Work out the finished part from the listing and answer in its coordinate system (mm). Round coordinates to 2 decimals unless told otherwise and drop trailing zeros. Answer in a Markdown table with one row per item.
```python
from build123d import *

# Parameters (mm, degrees)
MOTOR_AND_BATTERY_FLOOR_PROFILE_R   = 2.75
MOTOR_AND_BATTERY_FLOOR_PROFILE_R_2 = 1.75
MOTOR_AND_BATTERY_FLOOR_PROFILE_R_3 = 2.2
MOTOR_AND_BATTERY_FLOOR_DEPTH       = 2


with BuildPart() as part:
    # Motor and battery floor profile → Motor and battery floor (new body)
    with BuildSketch(Plane.XY):
        Polygon((-140, -143), (-94, -143), (-94, -104), (93, -104), (93, -143), (103, -143), (103, 143), (93, 143), (93, 104), (-94, 104), (-94, 143), (-140, 143), align=None)
        with Locations((-90, -91)):
            Circle(MOTOR_AND_BATTERY_FLOOR_PROFILE_R, mode=Mode.SUBTRACT)
        with Locations((-90, 91)):
            Circle(MOTOR_AND_BATTERY_FLOOR_PROFILE_R, mode=Mode.SUBTRACT)
        with Locations((-31, -91)):
            Circle(MOTOR_AND_BATTERY_FLOOR_PROFILE_R, mode=Mode.SUBTRACT)
        with Locations((-31, 91)):
            Circle(MOTOR_AND_BATTERY_FLOOR_PROFILE_R, mode=Mode.SUBTRACT)
        with Locations((31, -91)):
            Circle(MOTOR_AND_BATTERY_FLOOR_PROFILE_R, mode=Mode.SUBTRACT)
        with Locations((31, 91)):
            Circle(MOTOR_AND_BATTERY_FLOOR_PROFILE_R, mode=Mode.SUBTRACT)
        with Locations((90, -91)):
            Circle(MOTOR_AND_BATTERY_FLOOR_PROFILE_R, mode=Mode.SUBTRACT)
        with Locations((90, 91)):
            Circle(MOTOR_AND_BATTERY_FLOOR_PROFILE_R, mode=Mode.SUBTRACT)
        with Locations((-134, -108)):
            Circle(MOTOR_AND_BATTERY_FLOOR_PROFILE_R_2, mode=Mode.SUBTRACT)
        with Locations((-134, -17)):
            Circle(MOTOR_AND_BATTERY_FLOOR_PROFILE_R_2, mode=Mode.SUBTRACT)
        with Locations((-134, 17)):
            Circle(MOTOR_AND_BATTERY_FLOOR_PROFILE_R_2, mode=Mode.SUBTRACT)
        with Locations((-134, 108)):
            Circle(MOTOR_AND_BATTERY_FLOOR_PROFILE_R_2, mode=Mode.SUBTRACT)
        with Locations((-98, -108)):
            Circle(MOTOR_AND_BATTERY_FLOOR_PROFILE_R_2, mode=Mode.SUBTRACT)
        with Locations((-98, -17)):
            Circle(MOTOR_AND_BATTERY_FLOOR_PROFILE_R_2, mode=Mode.SUBTRACT)
        with Locations((-98, 17)):
            Circle(MOTOR_AND_BATTERY_FLOOR_PROFILE_R_2, mode=Mode.SUBTRACT)
        with Locations((-98, 108)):
            Circle(MOTOR_AND_BATTERY_FLOOR_PROFILE_R_2, mode=Mode.SUBTRACT)
        with Locations((-89, -46)):
            Circle(MOTOR_AND_BATTERY_FLOOR_PROFILE_R_2, mode=Mode.SUBTRACT)
        with Locations((-89, 46)):
            Circle(MOTOR_AND_BATTERY_FLOOR_PROFILE_R_2, mode=Mode.SUBTRACT)
        with Locations((-47, -46)):
            Circle(MOTOR_AND_BATTERY_FLOOR_PROFILE_R_2, mode=Mode.SUBTRACT)
        with Locations((-47, 46)):
            Circle(MOTOR_AND_BATTERY_FLOOR_PROFILE_R_2, mode=Mode.SUBTRACT)
        with Locations((-27, -46)):
            Circle(MOTOR_AND_BATTERY_FLOOR_PROFILE_R_2, mode=Mode.SUBTRACT)
        with Locations((-27, 46)):
            Circle(MOTOR_AND_BATTERY_FLOOR_PROFILE_R_2, mode=Mode.SUBTRACT)
        with Locations((15, -46)):
            Circle(MOTOR_AND_BATTERY_FLOOR_PROFILE_R_2, mode=Mode.SUBTRACT)
        with Locations((15, 46)):
            Circle(MOTOR_AND_BATTERY_FLOOR_PROFILE_R_2, mode=Mode.SUBTRACT)
        with Locations((35, -46)):
            Circle(MOTOR_AND_BATTERY_FLOOR_PROFILE_R_2, mode=Mode.SUBTRACT)
        with Locations((35, 46)):
            Circle(MOTOR_AND_BATTERY_FLOOR_PROFILE_R_2, mode=Mode.SUBTRACT)
        with Locations((77, -46)):
            Circle(MOTOR_AND_BATTERY_FLOOR_PROFILE_R_2, mode=Mode.SUBTRACT)
        with Locations((77, 46)):
            Circle(MOTOR_AND_BATTERY_FLOOR_PROFILE_R_2, mode=Mode.SUBTRACT)
        with Locations((-117, -135)):
            Circle(MOTOR_AND_BATTERY_FLOOR_PROFILE_R, mode=Mode.SUBTRACT)
        with Locations((-117, 135)):
            Circle(MOTOR_AND_BATTERY_FLOOR_PROFILE_R, mode=Mode.SUBTRACT)
        with Locations((98, -135)):
            Circle(MOTOR_AND_BATTERY_FLOOR_PROFILE_R, mode=Mode.SUBTRACT)
        with Locations((98, 135)):
            Circle(MOTOR_AND_BATTERY_FLOOR_PROFILE_R, mode=Mode.SUBTRACT)
        with Locations((98.5, -89)):
            Circle(MOTOR_AND_BATTERY_FLOOR_PROFILE_R, mode=Mode.SUBTRACT)
        with Locations((98.5, 0)):
            Circle(MOTOR_AND_BATTERY_FLOOR_PROFILE_R, mode=Mode.SUBTRACT)
        with Locations((98.5, 89)):
            Circle(MOTOR_AND_BATTERY_FLOOR_PROFILE_R, mode=Mode.SUBTRACT)
        with Locations((-134, -130)):
            Circle(MOTOR_AND_BATTERY_FLOOR_PROFILE_R_3, mode=Mode.SUBTRACT)
        with Locations((-134, 0)):
            Circle(MOTOR_AND_BATTERY_FLOOR_PROFILE_R_3, mode=Mode.SUBTRACT)
        with Locations((-134, 130)):
            Circle(MOTOR_AND_BATTERY_FLOOR_PROFILE_R_3, mode=Mode.SUBTRACT)
        with Locations((-37, -81)):
            Circle(MOTOR_AND_BATTERY_FLOOR_PROFILE_R_3, mode=Mode.SUBTRACT)
        with Locations((-37, 81)):
            Circle(MOTOR_AND_BATTERY_FLOOR_PROFILE_R_3, mode=Mode.SUBTRACT)
        with Locations((30, -81)):
            Circle(MOTOR_AND_BATTERY_FLOOR_PROFILE_R_3, mode=Mode.SUBTRACT)
        with Locations((30, 81)):
            Circle(MOTOR_AND_BATTERY_FLOOR_PROFILE_R_3, mode=Mode.SUBTRACT)
        with Locations((-132, -115)):
            Circle(MOTOR_AND_BATTERY_FLOOR_PROFILE_R_2, mode=Mode.SUBTRACT)
        with Locations((-132, -5)):
            Circle(MOTOR_AND_BATTERY_FLOOR_PROFILE_R_2, mode=Mode.SUBTRACT)
        with Locations((-132, 5)):
            Circle(MOTOR_AND_BATTERY_FLOOR_PROFILE_R_2, mode=Mode.SUBTRACT)
        with Locations((-132, 115)):
            Circle(MOTOR_AND_BATTERY_FLOOR_PROFILE_R_2, mode=Mode.SUBTRACT)
        with Locations((-100, -115)):
            Circle(MOTOR_AND_BATTERY_FLOOR_PROFILE_R_2, mode=Mode.SUBTRACT)
        with Locations((-100, -5)):
            Circle(MOTOR_AND_BATTERY_FLOOR_PROFILE_R_2, mode=Mode.SUBTRACT)
        with Locations((-100, 5)):
            Circle(MOTOR_AND_BATTERY_FLOOR_PROFILE_R_2, mode=Mode.SUBTRACT)
        with Locations((-100, 115)):
            Circle(MOTOR_AND_BATTERY_FLOOR_PROFILE_R_2, mode=Mode.SUBTRACT)
    extrude(amount=MOTOR_AND_BATTERY_FLOOR_DEPTH)


solid = part.part
```
1. The part is cut by section A-A (z = 1.5). Count the separate pieces of the cut face and the enclosed holes in it, plus the area to 3 significant figures.
Calculated:
| item | result |
|---|---|
| separate pieces | 1 |
| enclosed holes | 50 |
| area | 54,200 mm² |
2. Consider line 1 along X through (y, z) = (-115, 1.4); line 2 along X through (y, z) = (-81.5, 0.75); line 3 along X through (y, z) = (-135, 1.1). Determine where each line is inside the solid, lowest interval first. Write a range as from..to.
Calculated:
| item | result |
|---|---|
| line 1 | x = -140..-133.75, -130.25..-101.75, -98.25..-94, 93..103 |
| line 2 | x = -140..-39.14, -34.86..27.86, 32.14..103 |
| line 3 | x = -140..-119.75, -114.25..-94, 93..95.25, 100.75..103 |
3. Given pin 1 (3.5 mm diameter, centred on x = 30, y = -81, fed in from -Z), flat-ended and moving along its own axis, determine where the tip first touches the part or whether it passes through.
Calculated:
| item | result |
|---|---|
| pin 1 | passes through |
